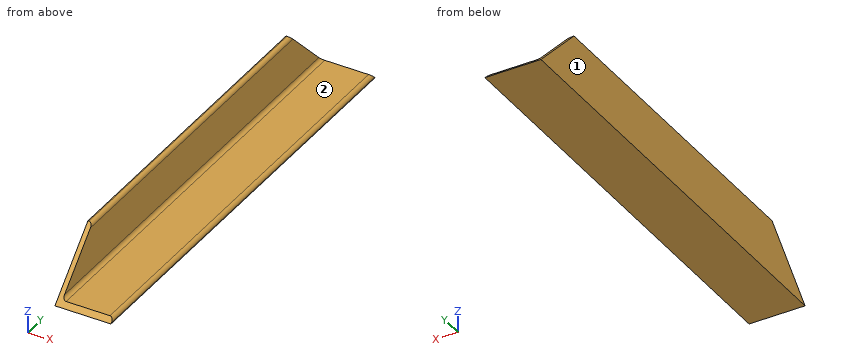
from build123d import *

# Parameters (mm, degrees)
F1_DEPTH = 304.8
F2_R     = 5.08
F4_DEPTH = 76.2


with BuildPart() as f1:
    # F0 (on Front) → F1 (new body, symmetric)
    with BuildSketch(Plane.XZ):
        Polygon((-38.1, -38.1), (38.1, -38.1), (38.1, -31.75), (-31.75, -31.75), (-31.75, 38.1), (-38.1, 38.1), align=None)
    extrude(amount=F1_DEPTH, both=True)

    # F2
    f2_edges = [f1.edges().sort_by_distance(p)[0] for p in [
        (-31.75, 0, 38.1),
        (-31.75, 0, -31.75),
        (38.1, 0, -31.75),
    ]]
    fillet(f2_edges, radius=F2_R)

    # F3 (on face) → F4 (cut)
    with BuildSketch(Plane(origin=(-38.1, 0, 0), x_dir=(0, -1, 0), z_dir=(-1, 0, 0))):
        Polygon((-304.8, 38.1), (-304.8, -38.1), (-228.6, 38.1), align=None)
        Polygon((228.6, 38.1), (304.8, -38.1), (304.8, 38.1), align=None)
    extrude(amount=-F4_DEPTH, mode=Mode.SUBTRACT)


solid = f1.part
Work out the finished part from the listing and answer in its coordinate system (mm). Face numbers are marked on the shaded views. A direction names the side the tool comes from. Round coordinates to 2 decimals unless told otherwise and drop trailing zeros. Order: outer loops, then holes, each group sorted by start corner. A loop starts at its lowest first (then second) coordinate and runs counter-clockwise, first axis right, second up. Notation, with made-up numbers: M 33.25,8 L 76.25,8 A37 cw 76.25,44 Z; hole C 46,57 d5. An arc over 180 degrees is marked long. Put each result on its own line as item: value. Start each with the question number.
Q1. Straight lines are drawn through the part: L1, parallel to X at y = 114, z = -19; L2, parallel to Z at x = -28, y = -138. For each, find the intervals that lie inside material, in ascending order. Write a range as [from, to].
Q2. Section D-D, the plane y = 21.5 is taken. Write down the section's boundary in (x, z), and give its area (3 significant figures).
Q3. A tool of negligible diameter and unlimited length cuts with its end or side. For the marked faces 1 and 2, from which of +Z, -Z, +X, -X, +Y, -Y can it reach the whole face along a straight path? Write none if from no direction.
Q4. Section C-C, the plane x = 2.5 is taken. Write down the section's boundary in (y, z), and give its area (3 significant figures).
Q5. Section B-B, the plane z = 8 is taken. Write down the section's boundary in (x, y), and give its area (3 significant figures).
Q6. A flat-ended cylindrical pin translates along its axis: pin 1 (18 mm diameter, centred on y = 14, z = -4, fed in from +X). Find the tip coordinate at first contact, or state that the pin passes through.
Q7. Section A-A, the plane y = 252 is taken. Write down the section's boundary in (x, z), and give its area (3 significant figures).
Findings below:
1. L1: x = [-38.1, -31.75]
1. L2: z = [-38.1, -31.57]
2. outline: M -38.1,-38.1 L 38.1,-38.1 L 38.1,-36.83 A5.08 ccw 33.02,-31.75 L -26.67,-31.75 A5.08 cw -31.75,-26.67 L -31.75,33.02 A5.08 ccw -36.83,38.1 L -38.1,38.1 Z
2. area: 922 mm^2
3. face 1: +Z, -Z, -X, +Y, -Y
3. face 2: +Z, +X, +Y, -Y
4. outline: M -304.8,-38.1 L 304.8,-38.1 L 298.45,-31.75 L -298.45,-31.75 Z
4. area: 3,830 mm^2
5. outline: M -38.1,-258.7 L -31.75,-258.7 L -31.75,258.7 L -38.1,258.7 Z
5. area: 3,290 mm^2
6. pin 1: stops at x = -31.75
7. outline: M -38.1,-38.1 L 38.1,-38.1 L 38.1,-36.83 A5.08 ccw 33.02,-31.75 L -26.67,-31.75 A5.08 cw -31.75,-26.67 L -31.75,14.7 L -38.1,14.7 Z
7. area: 779 mm^2
